Design review of the part built by this model. Coordinates are the model's own, in mm. A direction names the side the tool comes from. Round coordinates to 2 decimals unless told otherwise and drop trailing zeros. Loops run counter-clockwise (first coordinate to the right, second up) from the corner with the lowest first, then second, coordinate; pieces in that order, holes last. Notation, with made-up numbers: (81.25, 18.5) - (103.25, 18.5) arc R22 ccw to (103.25, 34.5) - close; hole circle Ø5 at (2.5, 22.5). An arc over 180 degrees is marked (long way). Use one line per item in the form item = value. Start each with the question number.
(1) We need section B-B, the plane z = 1. Write out the cut boundary in (x, y), then the cut area to 3 significant figures.
(2) The part is to be moulded in two halves that separate along X. For faces 4 (the flat face through (-5, 1, 5)), 5 (the flat face through (-1.146, -4.675, 0.023)), 6 (the cylindrical face through (-1.27, -0.97, 0.02)), say which applies: released by +X, released by -X, zero draft, split by the parting line, or undercut.
(3) For pin 1 (3 mm diameter, centred on y = 0, z = 3, fed in from +X); pin 2 (5 mm diameter, centred on x = 0, y = 0, fed in from -Z); pin 3 (3 mm diameter, centred on y = -2, z = -3, fed in from +X); pin 4 (1 mm diameter, centred on x = 0.5, y = -1.5, fed in from +Z), all flat-tipped, find the tip position at first contact; note any pin that passes through.
(4) We need section C-C, the plane x = -2.75. Write out the cut boundary in (y, z), then the cut area to 3 significant figures.
(5) We need section D-D, the plane z = -3. Write out the cut boundary in (x, y).
(6) Machinability: for faces 1 (the flat face through (-4, -2, -1.67)), 2 (the flat face through (-5, 1, -5)), 3 (the flat face through (-4.794, 0.035, 3.358)), which of the approach directions +Z, -Z, +X, -X, +Y, -Y give a long, thin tool a straight path to every point of the face, cutting with its end or side? Answer none if there is none.
(7) Wall thickness on probe 1 along X at (y, z) = (0, 0.95); probe 2 along Z at (x, y) = (-3.5, -2.75); probe 3 along Y at (x, z) = (-1.25, 1): over which ranges is each line inside the solid? List them lowest first. Write a range as [from, to].
(8) We need section A-A, the plane y = 0. Write out the cut boundary in (x, z), then the cut area to 3 significant figures.
from build123d import *

# Parameters (mm, degrees)
SKETCH1_R           = 1.6
BOSS_EXTRUDE1_DEPTH = 5
CUT_EXTRUDE2_DEPTH  = 3.33


with BuildPart() as part:
    # Sketch1 → Boss-Extrude1 (new body)
    with BuildSketch(Plane.XY):
        with BuildLine():
            Line((0, 2.5), (-7.5, 2.5))
            Line((-7.5, 2.5), (-7.5, -7.5))
            Line((-7.5, -7.5), (-3.976969112, -7.5))
            Line((-3.976969112, -7.5), (1.765839775, -1.769692032))
            ThreePointArc((1.765839775, -1.769692032), (2.310219695, 0.955450135), (0, 2.5))
        make_face()
        Circle(SKETCH1_R, mode=Mode.SUBTRACT)
    extrude(amount=BOSS_EXTRUDE1_DEPTH)

    # Sketch4 → Cut-Extrude2 (cut)
    with BuildSketch(Plane.XY.offset(5)):
        with BuildLine():
            Line((1.943040083, -1.946046052), (-3.82334364, -7.91054561))
            Line((-3.82334364, -7.91054561), (-8.510185697, -7.91054561))
            Line((-8.510185697, -7.91054561), (-8.510185697, -2.424183437))
            Line((-8.510185697, -2.424183437), (-2.010547232, 1.876219558))
            ThreePointArc((-2.010547232, 1.876219558), (1.911430852, 1.977101945), (1.943040083, -1.946046052))
        make_face()
    extrude(amount=-CUT_EXTRUDE2_DEPTH, mode=Mode.SUBTRACT)

    # Mirror1: part across plane


with BuildPart() as part_1:
    add(part.part)
    add(part.part.mirror(Plane.XY))


solid = part_1.part
Data:
q1.outline = (-7.5, -7.5) - (-3.98, -7.5) - (1.77, -1.77) arc R2.5 ccw to (0, 2.5) - (-7.5, 2.5) - close; hole circle Ø3.2 at (0, 0)
q1.area = 69.6 mm^2
q2.face_4 = zero draft
q2.face_5 = released by +X
q2.face_6 = undercut
q3.pin_1 = 2.5
q3.pin_2 = -1.67
q3.pin_3 = 2.13
q3.pin_4 = 1.67
q4.outline = (-6.28, -1.67) - (1.39, -1.67) - (1.39, -5) - (2.5, -5) - (2.5, 5) - (1.39, 5) - (1.39, 1.67) - (-6.28, 1.67) - close
q4.area = 36.7 mm^2
q5.outline = (-7.5, -1.76) - (-2.01, 1.88) arc R2.75 cw to (-1.15, 2.5) - (-7.5, 2.5) - close
q6.face_1 = -Z, +X, -Y
q6.face_2 = -Z, +X, -X, +Y, -Y
q6.face_3 = +Z, +X, -Y
q7.probe_1 = [-7.5, -1.6], [1.6, 2.5]
q7.probe_2 = [-1.67, 1.67]
q7.probe_3 = [-4.78, -1], [1, 2.5]
q8.outline = (-7.5, -5) - (-4.85, -5) - (-4.85, -1.67) - (-1.6, -1.67) - (-1.6, 1.67) - (-4.85, 1.67) - (-4.85, 5) - (-7.5, 5) - close; (1.6, -1.67) - (2.5, -1.67) - (2.5, 1.67) - (1.6, 1.67) - close
q8.area = 40.4 mm^2
